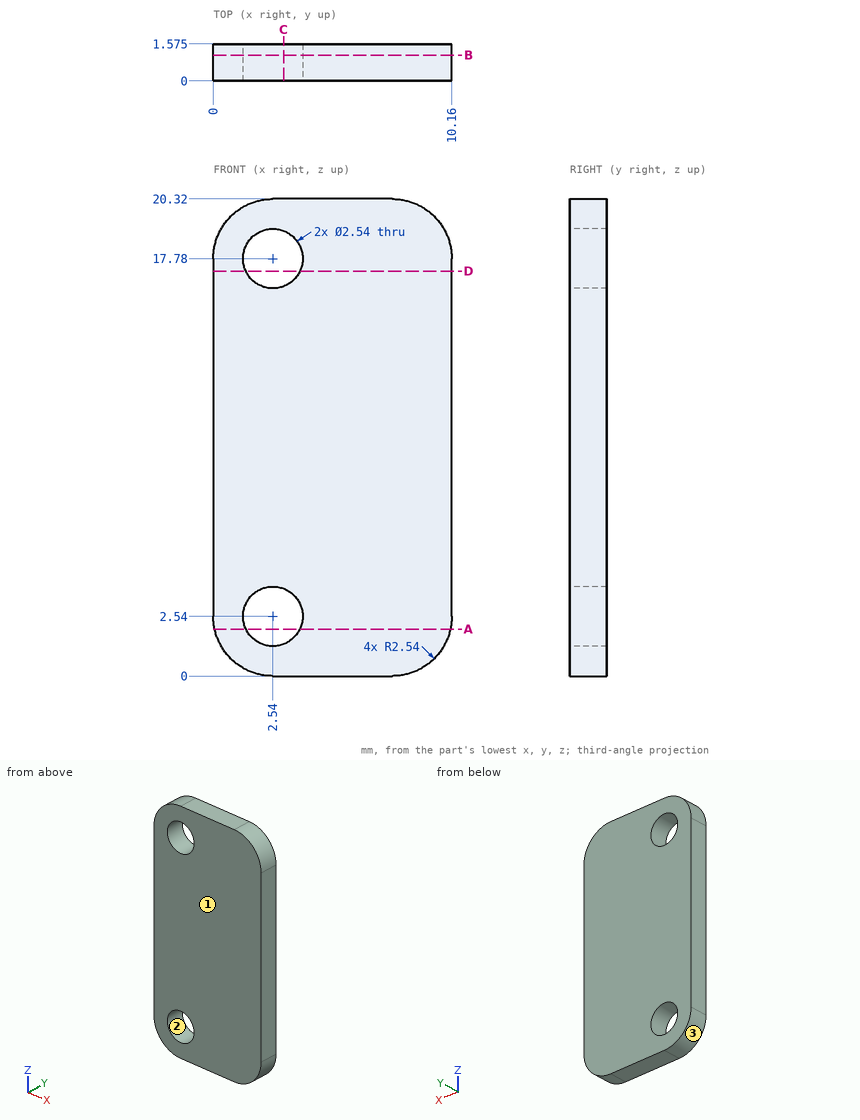
The figure shows three views and two pictorial views of one solid part (mm, origin at its lowest corner). Answer the questions. Give positions to 0.01 mm unless a question says otherwise; leave off trailing zeros. Loops run counter-clockwise (first coordinate to the right, second up) from the corner with the lowest first, then second, coordinate; pieces in that order, holes last. Notation, with made-up numbers: (43.5, 7.5) -> (68.5, 7.5) arc R20 ccw to (68.5, 25.5) -> close; hole circle Ø8 at (-8.75, 59.25). An arc over 180 degrees is marked (long way). Use CSV: the item, a comma, the result in double quotes.
1. The part is cut by section C-C (x = 3). Write down the section's boundary in (y, z) (1 decimal).
Found:
outline,"(0, 0) -> (1.6, 0) -> (1.6, 1.4) -> (0, 1.4) -> close; (0, 3.7) -> (1.6, 3.7) -> (1.6, 16.6) -> (0, 16.6) -> close; (0, 19) -> (1.6, 19) -> (1.6, 20.3) -> (0, 20.3) -> close"
2. Straight lines are drawn through the part: line 1 (Z direction, x = 2.54, y = 0.95); line 2 (Z direction, x = 3.25, y = 0.2); line 3 (X direction, y = 0.7, z = 17.25). For each, find the intervals that lie inside material, in ascending order.
Found:
line 1,"0 to 1.27, 3.81 to 16.51, 19.05 to 20.32"
line 2,"0 to 1.49, 3.59 to 16.73, 18.83 to 20.32"
line 3,"0 to 1.39, 3.69 to 10.16"
3. The mould has two halves that part along Z. Classify the marked faces 1, 2 and 3: +Z half, -Z half, draft (parallel to the pull), parting line (faces both ways), or undercut.
Found:
face 1,"draft"
face 2,"undercut"
face 3,"-Z half"
4. The part is cut by section D-D (z = 17.25). Write down the section's boundary in (x, y) (1 decimal), then the cut area to 3 significant figures.
Found:
outline,"(0, 0) -> (1.4, 0) -> (1.4, 1.6) -> (0, 1.6) -> close; (3.7, 0) -> (10.2, 0) -> (10.2, 1.6) -> (3.7, 1.6) -> close"
area,"12.4 mm^2"
5. The part is cut by section A-A (z = 2). Write down the section's boundary in (x, y) (1 decimal).
Found:
outline,"(0.1, 0) -> (1.4, 0) -> (1.4, 1.6) -> (0.1, 1.6) -> close; (3.7, 0) -> (10.1, 0) -> (10.1, 1.6) -> (3.7, 1.6) -> close"
6. The part is cut by section B-B (y = 1.1). Write down the section's boundary in (x, z).
Found:
outline,"(0, 2.54) arc R2.54 ccw to (2.54, 0) -> (7.62, 0) arc R2.54 ccw to (10.16, 2.54) -> (10.16, 17.78) arc R2.54 ccw to (7.62, 20.32) -> (2.54, 20.32) arc R2.54 ccw to (0, 17.78) -> close; hole circle Ø2.54 at (2.54, 2.54); hole circle Ø2.54 at (2.54, 17.78)"
7. Flat-ended cylindrical pins translate along their axes: pin 1 Ø1.5 at (x, z) = (2.54, 17.78) entering from -Y; pin 2 Ø4 at (x, z) = (5.5, 7) entering from -Y. Find the tip coordinate at first contact, or state that the pin passes through.
Found:
pin 1,"through"
pin 2,"y = 0"
